The figure shows three views and two pictorial views of one solid part (mm, origin at its lowest corner). Answer the questions. A direction names the side the tool comes from. Coordinates: 2 decimals unless noted, no trailing zeros. Order: outer loops, then holes, each group sorted by start corner. A loop starts at its lowest first (then second) coordinate and runs counter-clockwise, first axis right, second up. Notation, with made-up numbers: (1.5, -25.5) - (14.5, -25.5) arc R12 cw to (14.5, -16.5) - close; hole circle Ø10 at (-23, -33). An arc over 180 degrees is marked (long way). Use one line per item in the form item = value. Start each with the question number.
Item 1: Section A-A, the plane y = 15 is taken. Write down the section's boundary in (x, z).
Item 2: The mould has two halves that part along X. Classify the marked faces 1, 2 and 3: released by +X, released by -X, zero draft, split by the parting line, or undercut.
Item 3: Section C-C, the plane x = 9.5 is taken. Write down the section's boundary in (y, z).
Item 4: Consider line 1 along Z through (x, y) = (0.95, 21); line 2 along X through (y, z) = (8.75, 17); line 3 along X through (y, z) = (21.75, 12). Determine where each line is inside the solid, lowest interval first. Write a range as [from, to].
Item 5: Section B-B, the plane z = 18 is taken. Count the separate pieces of the cut face and the enclosed holes in it, and give its area (3 significant figures).
Item 6: Each of these flat-tipped pins is pushed along its axis until it touches: pin 1 Ø2.5 at (y, z) = (3, 33) entering from +X; pin 2 Ø6 at (x, y) = (12, 13.5) entering from +Z; pin 3 Ø2 at (x, y) = (13, 17) entering from -Z. Where does it stop, or does it pass through?
Item 7: Section D-D, the plane z = 14 is taken. Write down the section's boundary in (x, y), and give its area (3 significant figures).
Item 8: A tool of negligible diameter and unlimited length cuts with its end or side. For the marked faces 4, 5 and 6, from which of +Z, -Z, +X, -X, +Y, -Y can it reach the whole face along a straight path? Write none if from no direction.
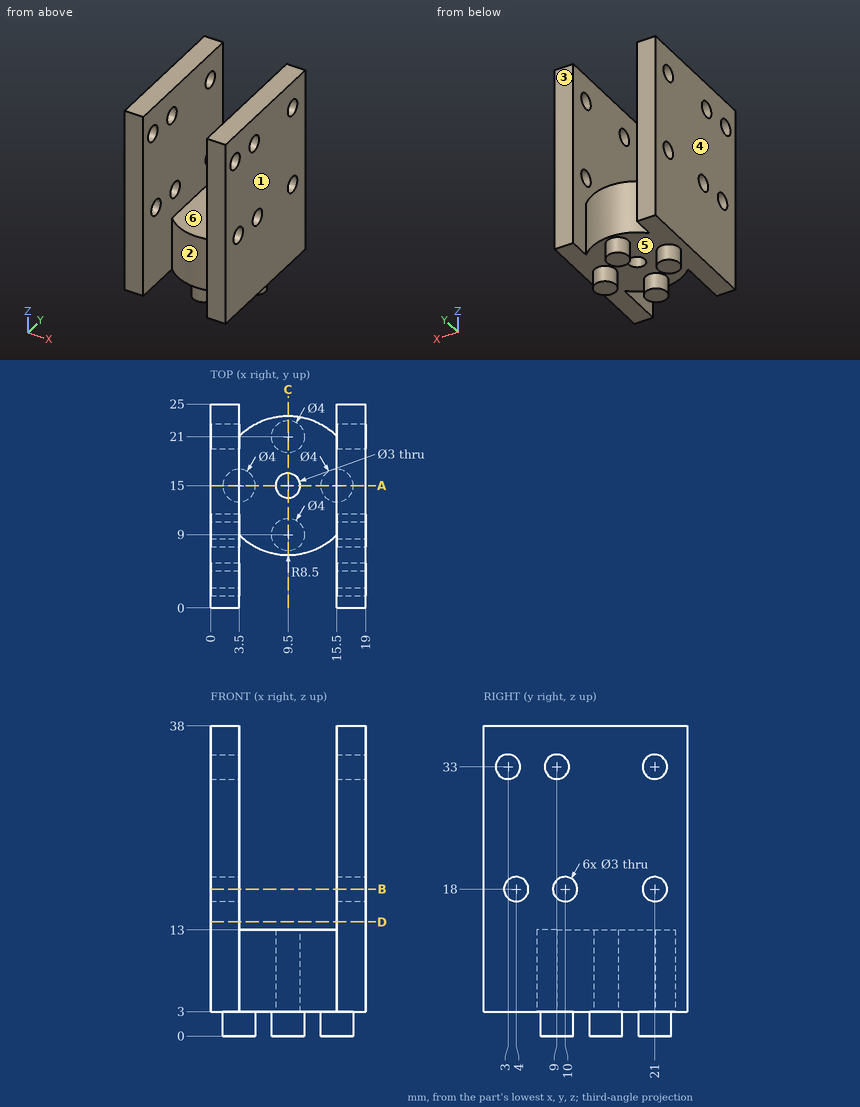
Response:
q1.outline = (0, 3) - (1.5, 3) - (1.5, 0) - (5.5, 0) - (5.5, 3) - (8, 3) - (8, 13) - (3.5, 13) - (3.5, 38) - (0, 38) - close; (11, 3) - (13.5, 3) - (13.5, 0) - (17.5, 0) - (17.5, 3) - (19, 3) - (19, 38) - (15.5, 38) - (15.5, 13) - (11, 13) - close
q2.face_1 = released by +X
q2.face_2 = undercut
q2.face_3 = zero draft
q3.outline = (6.5, 3) - (7, 3) - (7, 0) - (11, 0) - (11, 3) - (13.5, 3) - (13.5, 13) - (6.5, 13) - close; (16.5, 3) - (19, 3) - (19, 0) - (23, 0) - (23, 3) - (23.5, 3) - (23.5, 13) - (16.5, 13) - close
q4.line_1 = [3, 16.5], [19.5, 31.5], [34.5, 38]
q4.line_2 = [0, 3.5], [15.5, 19]
q4.line_3 = [0, 3.5], [4.33, 14.67], [15.5, 19]
q5.separate_pieces = 8
q5.enclosed_holes = 0
q5.area = 112 mm2
q6.pin_1 = through
q6.pin_2 = 13
q6.pin_3 = 3
q7.outline = (0, 0) - (3.5, 0) - (3.5, 25) - (0, 25) - close; (15.5, 0) - (19, 0) - (19, 25) - (15.5, 25) - close
q7.area = 175 mm2
q8.face_4 = +Z, -Z, -X, +Y, -Y
q8.face_5 = -Z
q8.face_6 = +Z, +Y, -Y
